from build123d import *

# Parameters (mm, degrees)
F0_W     = 20
F0_H     = 120
F1_DEPTH = 5
F2_R     = 3
F3_DEPTH = 5.001
F5_D     = 6
F6_SIZE  = 0.5
F7_R     = 5


with BuildPart() as f1:
    # F0 (on Front) → F1 (new body)
    with BuildSketch(Plane.XZ):
        with Locations((10, 60)):
            Rectangle(F0_W, F0_H)
    extrude(amount=F1_DEPTH)

    # F2 (on face) → F3 (cut, through all)
    with BuildSketch(Plane.XZ.offset(5)):
        with Locations((10, 110)):
            Circle(F2_R)
    extrude(amount=-F3_DEPTH, mode=Mode.SUBTRACT)

    # F5 (through all)
    with Locations(Plane.XZ.offset(5)):
        with Locations((10, 10)):
            Hole(F5_D / 2)

    # F6
    f6_edges = [f1.edges().sort_by_distance(p)[0] for p in [
        (7, -5, 110),
        (7, 0, 110),
        (7, 0, 10),
        (7, -5, 10),
    ]]
    chamfer(f6_edges, length=F6_SIZE)

    # F7
    f7_edges = [f1.edges().sort_by_distance(p)[0] for p in [
        (20, -2.5, 120),
        (0, -2.5, 120),
        (20, -2.5, 0),
        (0, -2.5, 0),
    ]]
    fillet(f7_edges, radius=F7_R)


solid = f1.part
Input: part model. Units: mm. Frame: model coordinates. Coordinates: 2 decimals unless noted, no trailing zeros. Loops run counter-clockwise (first coordinate to the right, second up) from the corner with the lowest first, then second, coordinate; pieces in that order, holes last.
Q1. Contact query for a flat-ended pin moving along its axis: pin 1 (9.5 mm diameter, centred on x = 10, z = 10, fed in from +Y). Output: stop coordinate, or through.
Q2. Cut plane B-B (z = 110). Output: boundary loops of the cut face in (x, y).
Q3. Cut plane A-A (x = 10). Output: boundary loops of the cut face in (y, z), then the cut area to 3 significant figures.
Q4. Cut plane D-D (x = 18.5). Output: boundary loops of the cut face in (y, z).
Q5. Draft query along Z for faces 1 (the face through (10, -5, 61)), 2 (the face through (18, -3, 1)), 3 (the face through (12.86, -2.53, 110.9)). Return one class per face: +Z half, -Z half, draft (parallel to the pull), parting line (faces both ways), or undercut.
Q6. Cut plane C-C (y = -2.85). Output: boundary loops of the cut face in (x, z), then the cut area to 3 significant figures.
Q7. Material intervals for line 1 (Z direction, x = 10, y = -1.4); line 2 (Z direction, x = 7.75, y = -3.1); line 3 (Z direction, x = 1, y = -3.45), sorted ascending.
Working result:
1. pin 1: stops at y = 0
2. outline: (0, -5) - (6.5, -5) - (7, -4.5) - (7, -0.5) - (6.5, 0) - (0, 0) - close; (13, -4.5) - (13.5, -5) - (20, -5) - (20, 0) - (13.5, 0) - (13, -0.5) - close
3. outline: (-5, 0) - (0, 0) - (0, 6.5) - (-0.5, 7) - (-4.5, 7) - (-5, 6.5) - close; (-5, 13.5) - (-4.5, 13) - (-0.5, 13) - (0, 13.5) - (0, 106.5) - (-0.5, 107) - (-4.5, 107) - (-5, 106.5) - close; (-5, 113.5) - (-4.5, 113) - (-0.5, 113) - (0, 113.5) - (0, 120) - (-5, 120) - close
3. area: 539 mm2
4. outline: (-5, 1.43) - (0, 1.43) - (0, 118.57) - (-5, 118.57) - close
5. face 1: draft
5. face 2: -Z half
5. face 3: undercut
6. outline: (0, 5) arc R5 ccw to (5, 0) - (15, 0) arc R5 ccw to (20, 5) - (20, 115) arc R5 ccw to (15, 120) - (5, 120) arc R5 ccw to (0, 115) - close; hole circle Ø6 at (10, 10); hole circle Ø6 at (10, 110)
6. area: 2,320 mm2
7. line 1: z = 0 to 7, 13 to 107, 113 to 120
7. line 2: z = 0 to 8.02, 11.98 to 108.02, 111.98 to 120
7. line 3: z = 2 to 118
